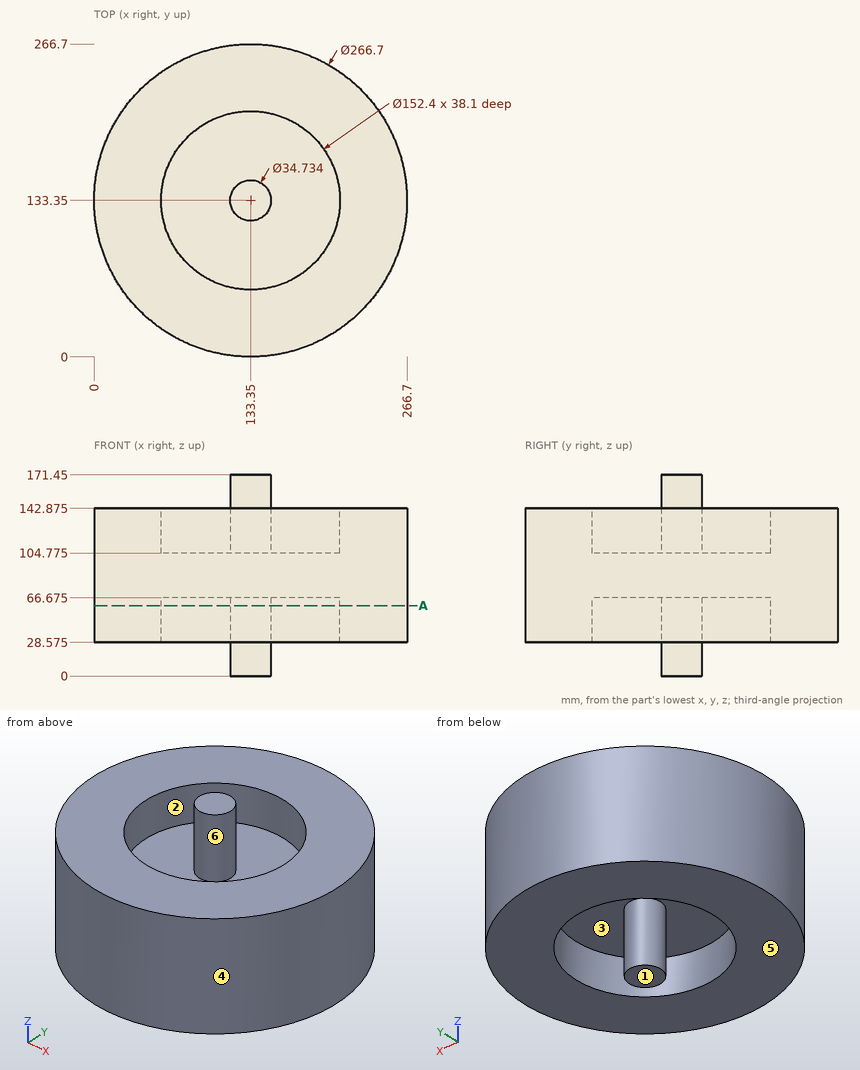
Source: three-view drawing plus pictorial views. Frame: mm from the lowest corner of the part. A direction names the side the tool comes from. Round coordinates to 2 decimals unless told otherwise and drop trailing zeros. Use one line per item in the form item = value. Start each with the question number.
1. Line query: probe 1 along Y at (x, z) = (133, 115); probe 2 along Z at (x, y) = (69, 236) (1 decimal). Output: solid intervals per line, ascending.
2. Draft query along Y for the marked faces 4, 5 and 6. Return one class per face: pulls with the +Y half, pulls with the -Y half, needs draft (parallel to the pull), parting line crosses it, or undercut.
3. Cut plane A-A (z = 60). Count the separate pieces of the cut face and the enclosed holes in it, then the cut area to 3 significant figures.
4. Pin query (flat end, axial travel): pin 1 Ø12 at (x, y) = (141, 235) entering from -Z (1 decimal); pin 2 Ø1 at (y, z) = (35, 60) entering from -X (1 decimal); pin 3 Ø8 at (y, z) = (143, 111.5) entering from +X. Return the tip coordinate at first contact, or that it passes through.
5. Reachability of the marked faces 1, 2 and 3 from +Z, -Z, +X, -X, +Y, -Y: full face, straight path, thin tool, end or side. Return the list, or none.
Solution:
q1.probe_1 = 0 to 57.15, 115.99 to 150.71, 209.55 to 266.7
q1.probe_2 = 28.6 to 142.9
q2.face_4 = parting line crosses it
q2.face_5 = needs draft
q2.face_6 = undercut
q3.separate_pieces = 2
q3.enclosed_holes = 1
q3.area = 38,600 mm^2
q4.pin_1 = 28.6
q4.pin_2 = 42.8
q4.pin_3 = 266.58
q5.face_1 = -Z, +X, -X, +Y, -Y
q5.face_2 = +Z
q5.face_3 = -Z
